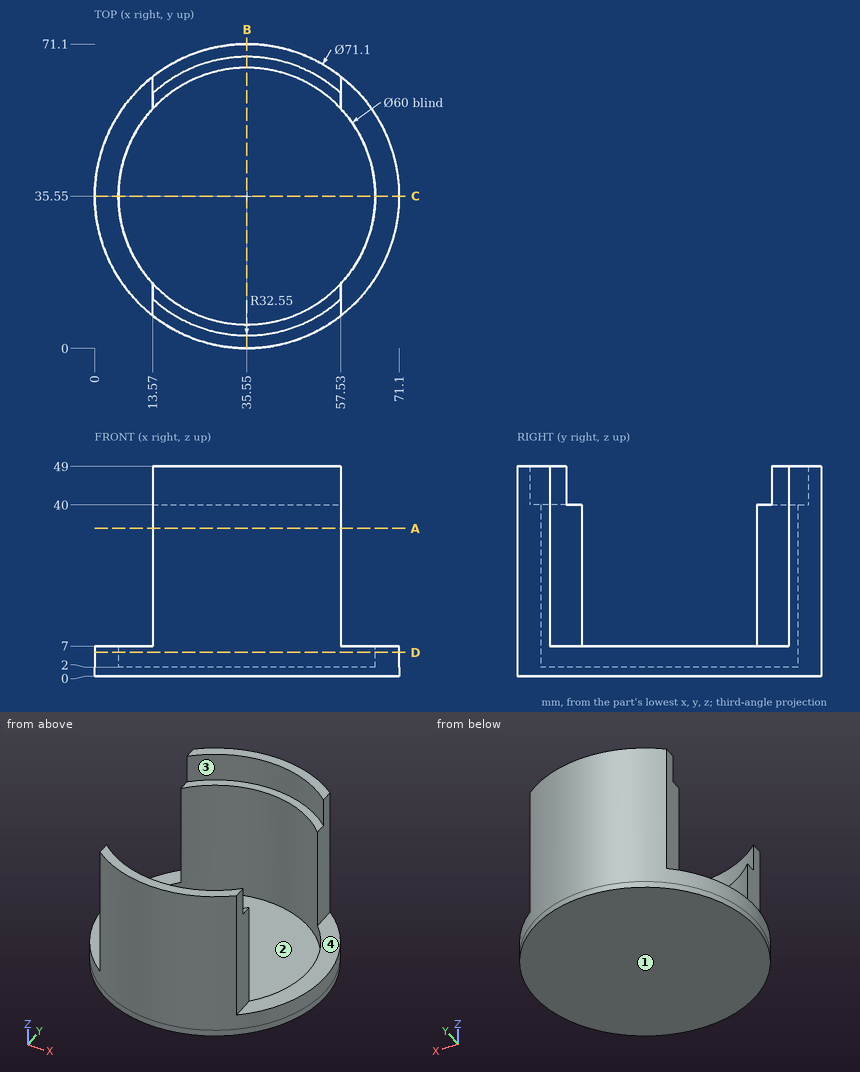
Could you check a few things on this drawing? It's one solid part, dimensions in mm from its lowest x, y, z. A direction names the side the tool comes from. Round coordinates to 2 decimals unless told otherwise and drop trailing zeros. Loops run counter-clockwise (first coordinate to the right, second up) from the corner with the lowest first, then second, coordinate; pieces in that order, holes last. Notation, with made-up numbers: M -32.75,57.25 L -24.75,57.25 A27 ccw -24.75,94.25 Z; hole C 46,75 d5. An arc over 180 degrees is marked long. Write each question's results on one line, items separated by ' | '. Start each with the question number.
(1) Thinking about a two-plate mould opening in X: for the marked faces 1 and 2, which applies, pulls with the +X half, pulls with the -X half, needs draft (parallel to the pull), parting line crosses it, or undercut?
(2) Will these pins go through, and if not, where does the flat tip stop? P1, Ø7, axis at x = 67, y = 24, coming from the +Z side; P2, Ø12, axis at y = 61.5, z = 19, coming from the -X side; P3, Ø4, axis at x = 33.5, z = 35.5, coming from the -Y side; P4, Ø10, axis at x = 47.5, y = 7.5, coming from the +Z side.
(3) I want a section at D-D (z = 5.5). Please give me the cut outline in (x, y), then the cut area to 3 significant figures.
(4) If I drill on probe 1 along Y at (x, z) = (35, 23) (3 decimals); probe 2 along Z at (x, y) = (41.5, 14); probe 3 along Z at (x, y) = (67.5, 40.5), over which ranges is the centre line in solid material (lowest first)? Write a range as from..to.
(5) I want a section at C-C (y = 35.55). Please give me the cut outline in (x, z).
(6) On a 3-axis mill with a long thin cutter (end or side, diameter ignored), from which of +Z, -Z, +X, -X, +Y, -Y can I reach the whole of each face in a straight line? I mean the marked faces 3 and 4. Say none if no direction works.
(7) I want a section at B-B (x = 35.55). Please give me the cut outline in (y, z).
(8) I want a section at A-A (z = 34.5). Please give me the cut outline in (x, y).
Solved:
1) face 1: needs draft | face 2: undercut
2) P1: stops at z = 7 | P2: stops at x = 13.57 | P3: stops at y = 0 | P4: stops at z = 49
3) outline: C 35.55,35.55 d71.1; hole C 35.55,35.55 d60 | area: 1,140 mm²
4) probe 1: y = 0.004..5.555, 65.545..71.096 | probe 2: z = 0..2 | probe 3: z = 0..7
5) outline: M 0,0 L 71.1,0 L 71.1,7 L 65.55,7 L 65.55,2 L 5.55,2 L 5.55,7 L 0,7 Z
6) face 3: +Z | face 4: +Z, +X, +Y, -Y
7) outline: M 0,0 L 71.1,0 L 71.1,49 L 68.1,49 L 68.1,40 L 65.55,40 L 65.55,2 L 5.55,2 L 5.55,40 L 3,40 L 3,49 L 0,49 Z
8) outline: M 13.57,7.61 A35.55 ccw 57.53,7.61 L 57.53,15.13 A30 cw 13.57,15.13 Z; M 13.57,55.97 A30 cw 57.53,55.97 L 57.53,63.49 A35.55 ccw 13.57,63.49 Z
